Study the drawing (mm; zero at the part's minimum x, y, z) and answer. A direction names the side the tool comes from. Coordinates: 2 decimals unless noted, no trailing zeros. Write each loop counter-clockwise with the first axis right and the second up, starting at its lowest first coordinate (ties: lowest second). Pieces come first, ordered by that corner, then holes. Notation, with made-up numbers: (-33.75, 23.5) -> (25.25, 23.5) arc R25 cw to (25.25, 48.5) -> close; hole circle Ø4 at (6, -1.5). An arc over 180 degrees is marked (long way). Write item = value, one per line. Start each with the question number.
1) Section A-A (z = 15.5) is taken. Determine the outline of the cut face in (x, y), plus the area to 3 significant figures.
2) For a pull along X with two mould halves and no side action, classify the marked faces 3, 4 and 5 as released by +X, released by -X, zero draft, split by the parting line, or undercut.
3) A tool of negligible diameter and unlimited length cuts with its end or side. For the marked faces 1 and 2, from which of +Z, -Z, +X, -X, +Y, -Y can it reach the whole face along a straight path? Write none if from no direction.
4) Section D-D (z = 4) is taken. Determine the outline of the cut face in (x, y), plus the area to 3 significant figures.
5) Flat-ended cylindrical pins translate along their axes: pin 1 Ø1.5 at (y, z) = (8.5, 4.5) entering from -X; pin 2 Ø1.5 at (x, y) = (11.5, 12) entering from +Z. Find the tip coordinate at first contact, or state that the pin passes through.
6) Section B-B (y = 28) is taken. Determine the outline of the cut face in (x, z).
7) Section C-C (x = 16.75) is taken. Determine the outline of the cut face in (y, z), plus the area to 3 significant figures.
8) Find the intervals of material crossed by line 1 along Y through (x, z) = (7.5, 4); line 2 along Z through (x, y) = (12.5, 8); line 3 along X through (y, z) = (29, 13), in increasing order. Write a range as from..to.
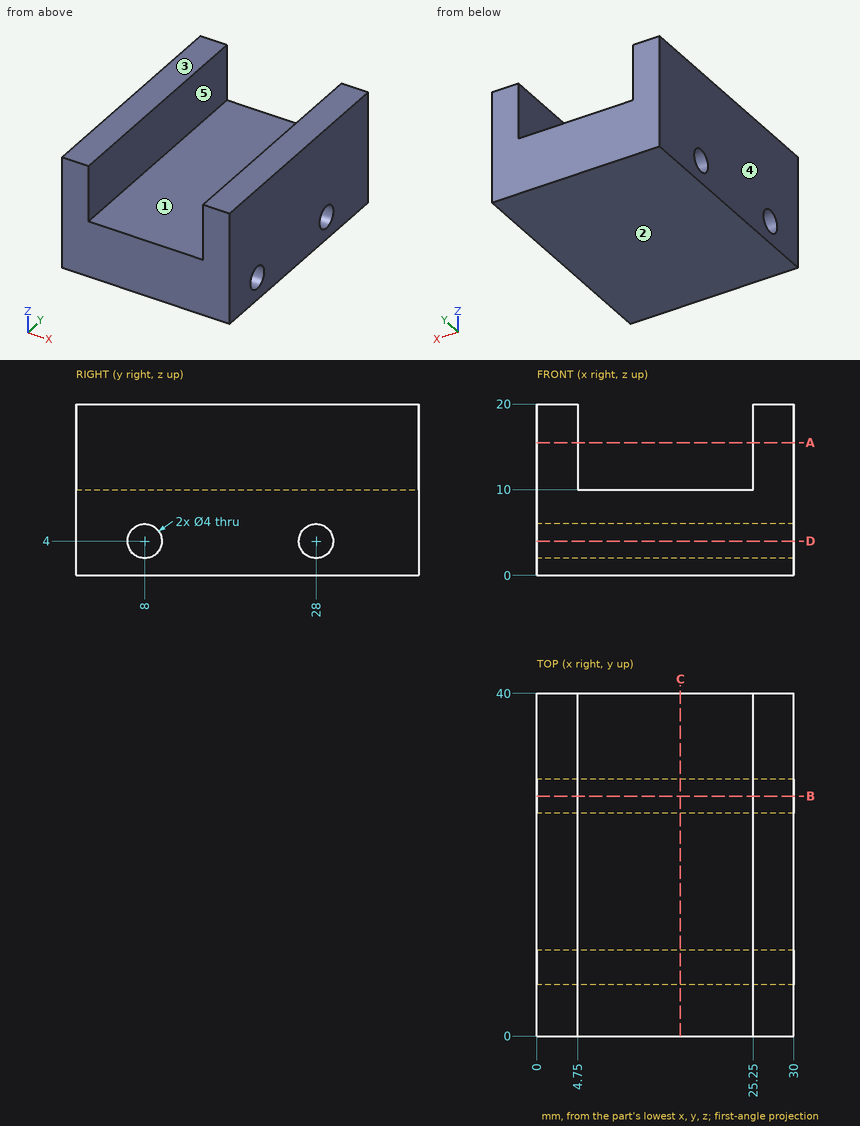
Answer key:
q1.outline = (0, 0) -> (4.75, 0) -> (4.75, 40) -> (0, 40) -> close; (25.25, 0) -> (30, 0) -> (30, 40) -> (25.25, 40) -> close
q1.area = 380 mm^2
q2.face_3 = zero draft
q2.face_4 = released by -X
q2.face_5 = undercut
q3.face_1 = +Z, +Y, -Y
q3.face_2 = -Z, +X, -X, +Y, -Y
q4.outline = (0, 0) -> (30, 0) -> (30, 6) -> (0, 6) -> close; (0, 10) -> (30, 10) -> (30, 26) -> (0, 26) -> close; (0, 30) -> (30, 30) -> (30, 40) -> (0, 40) -> close
q4.area = 960 mm^2
q5.pin_1 = through
q5.pin_2 = 10
q6.outline = (0, 0) -> (30, 0) -> (30, 2) -> (0, 2) -> close; (0, 6) -> (30, 6) -> (30, 20) -> (25.25, 20) -> (25.25, 10) -> (4.75, 10) -> (4.75, 20) -> (0, 20) -> close
q7.outline = (0, 0) -> (40, 0) -> (40, 10) -> (0, 10) -> close; hole circle Ø4 at (8, 4); hole circle Ø4 at (28, 4)
q7.area = 375 mm^2
q8.line_1 = 0..6, 10..26, 30..40
q8.line_2 = 0..2, 6..10
q8.line_3 = 0..4.75, 25.25..30
